Here's the drawing with two shaded views (mm, measured from the low corner). I have some questions. A direction names the side the tool comes from. Round coordinates to 2 decimals unless told otherwise and drop trailing zeros. Write each loop counter-clockwise with the first axis right and the second up, starting at its lowest first coordinate (ties: lowest second). Pieces come first, ordered by that corner, then holes. Notation, with made-up numbers: M 26.25,70.5 L 60.25,70.5 A17 ccw 60.25,102.5 Z; hole C 27,68 d8. An arc over 180 degrees is marked long. Use one line per item in the form item = value. Start each with the question number.
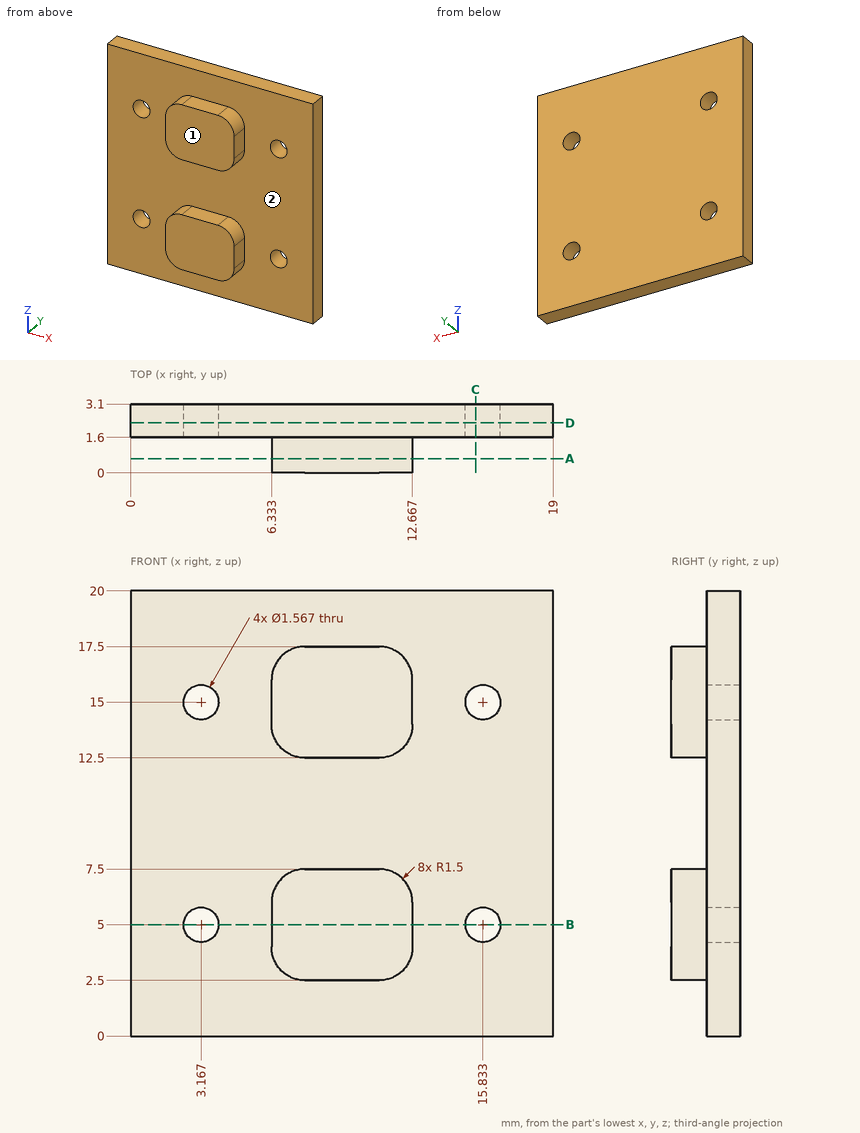
1. If we section it at B-B (z = 5): List the corners of the cut face in (x, y) for me.
2. If we section it at A-A (y = 0.65): List the corners of the cut face in (x, z) for me.
3. If we section it at C-C (x = 15.5): List the corners of the cut face in (y, z) for me.
4. Will these pins go through, and if not, where does the flat tip stop? pin 1 (2 mm diameter, centred on x = 3.17, z = 15, fed in from -Y); pin 2 (1.3 mm diameter, centred on y = 0.5, z = 5, fed in from -X); pin 3 (1.3 mm diameter, centred on x = 10, y = 0.5, fed in from -Z); pin 4 (1.4 mm diameter, centred on x = 3.17, z = 5, fed in from -Y).
5. Please list where these lines run through material, in increasing order: line 1 along X through (y, z) = (2.4, 15); line 2 along Z through (x, y) = (15.5, 1.7); line 3 along Z through (x, y) = (9, 0.4).
6. Which directions (+Z, -Z, +X, -X, +Y, -Y) give clear straight access to the entire face, cutting with the end or side of a thin tool? Please do the marked faces 1 and 2.
7. If we section it at D-D (y = 2.25): List the corners of the cut face in (x, z) for me, and give its area (3 significant figures).
Model answer:
q1.outline = M 0,1.6 L 2.38,1.6 L 2.38,3.1 L 0,3.1 Z; M 3.95,1.6 L 6.33,1.6 L 6.33,0 L 12.67,0 L 12.67,1.6 L 15.05,1.6 L 15.05,3.1 L 3.95,3.1 Z; M 16.62,1.6 L 19,1.6 L 19,3.1 L 16.62,3.1 Z
q2.outline = M 6.33,4 A1.5 ccw 7.83,2.5 L 11.17,2.5 A1.5 ccw 12.67,4 L 12.67,6 A1.5 ccw 11.17,7.5 L 7.83,7.5 A1.5 ccw 6.33,6 Z; M 6.33,14 A1.5 ccw 7.83,12.5 L 11.17,12.5 A1.5 ccw 12.67,14 L 12.67,16 A1.5 ccw 11.17,17.5 L 7.83,17.5 A1.5 ccw 6.33,16 Z
q3.outline = M 1.6,0 L 3.1,0 L 3.1,4.29 L 1.6,4.29 Z; M 1.6,5.71 L 3.1,5.71 L 3.1,14.29 L 1.6,14.29 Z; M 1.6,15.71 L 3.1,15.71 L 3.1,20 L 1.6,20 Z
q4.pin_1 = 1.6
q4.pin_2 = 6.33
q4.pin_3 = 2.5
q4.pin_4 = through
q5.line_1 = 0 to 2.38, 3.95 to 15.05, 16.62 to 19
q5.line_2 = 0 to 4.29, 5.71 to 14.29, 15.71 to 20
q5.line_3 = 2.5 to 7.5, 12.5 to 17.5
q6.face_1 = +Z, -Z, +X, -X, -Y
q6.face_2 = -Y
q7.outline = M 0,0 L 19,0 L 19,20 L 0,20 Z; hole C 3.17,5 d1.57; hole C 3.17,15 d1.57; hole C 15.83,5 d1.57; hole C 15.83,15 d1.57
q7.area = 372 mm2
